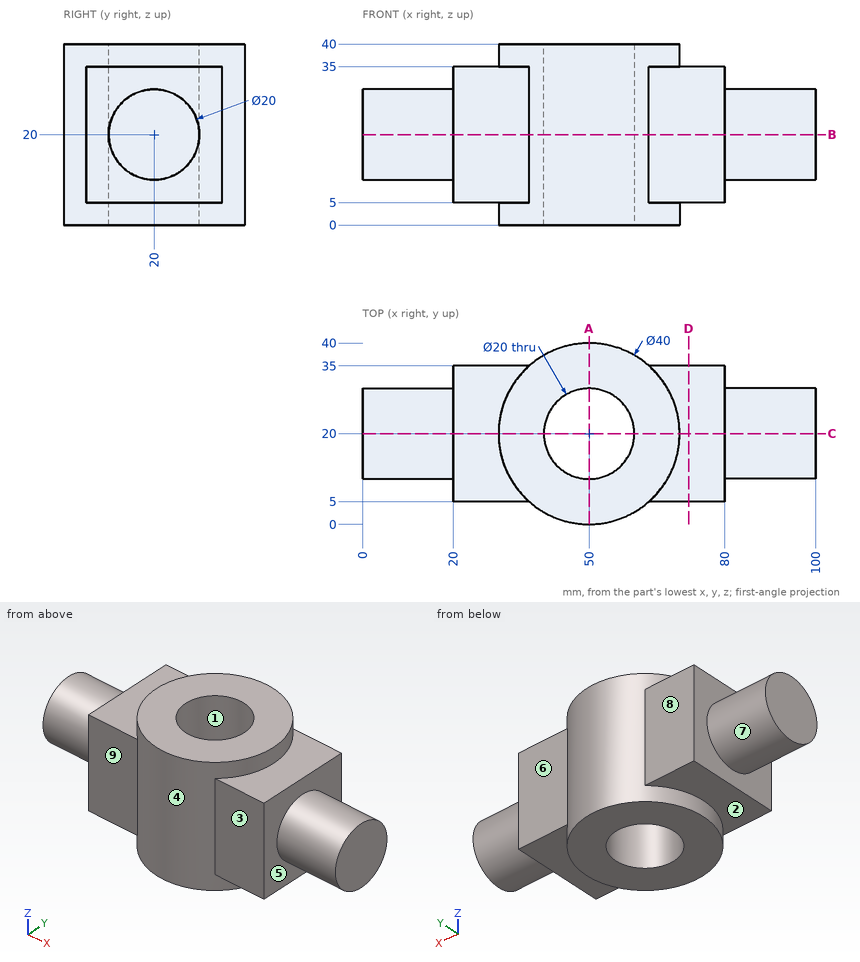
The drawing under review shows one solid part. Ordinate dimensions are in mm from its lowest x, y, z. A direction names the side the tool comes from. Give positions to 0.01 mm unless a question says otherwise; leave off trailing zeros. Write each loop counter-clockwise with the first axis right and the second up, starting at its lowest first coordinate (ties: lowest second). Pieces come first, ordered by that corner, then holes. Notation, with made-up numbers: (45, -9) - (71, -9) arc R13 cw to (71, 0) - close; hole circle Ø1 at (89.25, 71). An arc over 180 degrees is marked (long way). Answer in a Markdown table with one row per item. Add a question column.
1. We need section A-A on x = 50. Write out the cut boundary in (y, z).
2. Insertion check: P1, Ø13.5, axis at x = 76, y = 26.5, coming from the -Z side; P2, Ø1, axis at y = 16, z = 26, coming from the -X side; P3, Ø1, axis at x = 22.5, z = 21, coming from the +Y side; P4, Ø13.5, axis at x = 28, z = 20, coming from the -Y side. Each pin has a flat end and moves straight along its axis. Give the tip position at first contact, or say it passes through.
3. We need section D-D on x = 72. Write out the cut boundary in (y, z), then the cut area to 3 significant figures.
4. Wall thickness on line 1 along Y through (x, z) = (50, 17.5); line 2 along X through (y, z) = (20.5, 6); line 3 along Y through (x, z) = (26.5, 18.5): over which ranges is each line inside the solid? List them lowest first. Write a range as [from, to].
5. Tool access review of the marked faces 5, 6, 7, 8 and 9: name each direction out of +Z, -Z, +X, -X, +Y, -Y from which nothing blocks a thin tool from reaching the whole face with its end or side.
6. We need section C-C on y = 20. Write out the cut boundary in (x, z).
7. We need section B-B on z = 20. Write out the cut boundary in (x, y).
8. Draft analysis for pull direction Y (two halves, no side actions). For the marked faces 1, 2, 3 and 4, state which applies: +Y half, -Y half, draft (parallel to the pull), parting line (faces both ways), or undercut.
Ans:
| question | item | result |
|---|---|---|
| 1 | outline | (0, 0) - (10, 0) - (10, 40) - (0, 40) - close; (30, 0) - (40, 0) - (40, 40) - (30, 40) - close |
| 2 | P1 | stops at z = 5 |
| 2 | P2 | stops at x = 0 |
| 2 | P3 | stops at y = 35 |
| 2 | P4 | stops at y = 5 |
| 3 | outline | (5, 5) - (35, 5) - (35, 35) - (5, 35) - close |
| 3 | area | 900 mm^2 |
| 4 | line 1 | y = [0, 10], [30, 40] |
| 4 | line 2 | x = [20, 40.01], [59.99, 80] |
| 4 | line 3 | y = [5, 35] |
| 5 | face 5 | +X |
| 5 | face 6 | +Z, -Z, +X, +Y |
| 5 | face 7 | -X |
| 5 | face 8 | +Z, -Z, -X, +Y |
| 5 | face 9 | +Z, -Z, -X, -Y |
| 6 | outline | (0, 10) - (20, 10) - (20, 5) - (30, 5) - (30, 0) - (40, 0) - (40, 40) - (30, 40) - (30, 35) - (20, 35) - (20, 30) - (0, 30) - close; (60, 0) - (70, 0) - (70, 5) - (80, 5) - (80, 10) - (100, 10) - (100, 30) - (80, 30) - (80, 35) - (70, 35) - (70, 40) - (60, 40) - close |
| 7 | outline | (0, 10) - (20, 10) - (20, 5) - (36.77, 5) arc R20 ccw to (63.23, 5) - (80, 5) - (80, 10) - (100, 10) - (100, 30) - (80, 30) - (80, 35) - (63.23, 35) arc R20 ccw to (36.77, 35) - (20, 35) - (20, 30) - (0, 30) - close; hole circle Ø20 at (50, 20) |
| 8 | face 1 | undercut |
| 8 | face 2 | draft |
| 8 | face 3 | -Y half |
| 8 | face 4 | parting line |
